Could you check a few things on this model? Use its own coordinates, in mm. Face numbers are marked on the shaded views. A direction names the side the tool comes from. Give positions to 0.01 mm unless a question says otherwise; leave off trailing zeros. Loops run counter-clockwise (first coordinate to the right, second up) from the corner with the lowest first, then second, coordinate; pieces in that order, holes last. Notation, with made-up numbers: (10, 19) - (29, 19) arc R17 cw to (29, 35) - close; hole circle Ø3 at (1.25, 63). An arc over 180 degrees is marked (long way). Write each question's results on one line, items separated by ' | '. Start each with the question number.
1) I want a section at B-B, the plane z = 0. Write out the boundary of the cut face in (x, y), and give its area (3 significant figures).
2) I want a section at D-D, the plane y = -378. Write out the boundary of the cut face in (x, z).
3) I want a section at A-A, the plane y = 0. Write out the boundary of the cut face in (x, z).
4) On a 3-axis mill with a long thin cutter (end or side, diameter ignored), from which of +Z, -Z, +X, -X, +Y, -Y can I reach the whole of each face in a straight line? I mean the marked faces 1, 2, 3 and 4. Say none if no direction works.
5) I want a section at C-C, the plane y = 365. Write out the boundary of the cut face in (x, z).
6) If I drill on probe 1 along Z at (x, y) = (199, 0); probe 2 along Y at (x, z) = (177, 71); probe 3 along Z at (x, y) = (140.5, -277.5), over which ranges is the centre line in solid material (lowest first)? Write a range as [from, to].
7) I'm going to push flat-ended pins straight in: pin 1 (3 mm diameter, centred on x = 171.5, z = -234, fed in from +Y); pin 2 (2 mm diameter, centred on x = 47, z = -451, fed in from -Y); pin 3 (1.5 mm diameter, centred on x = 141.5, z = 200, fed in from +Y); pin 4 (8 mm diameter, centred on y = 408, z = -248.5, fed in from -X). Where does each tip first touch, or does it pass through?
8) If we mould it in two halves opening along Y, with no side actions, what happens to the marked faces 5, 6, 7 and 8? For each: +Y half, -Y half, draft (parallel to the pull), parting line (faces both ways), or undercut.
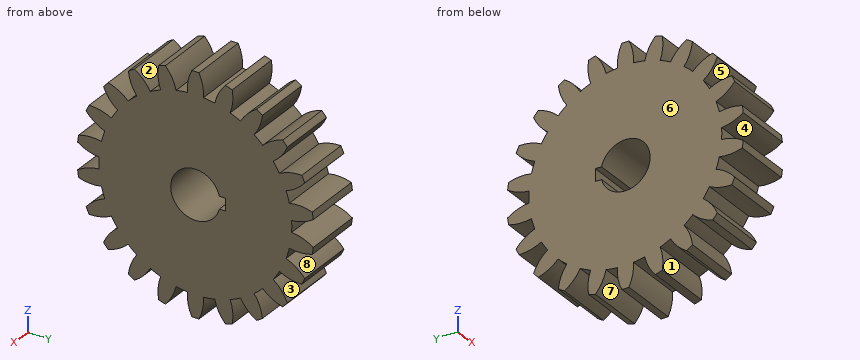
from build123d import *

# Parameters (mm, degrees)
BASPROSKE_W     = 304.8
BASPROSKE_H     = 609.6
TOOTHCUT_DEPTH  = 915.4
TEETHCUTS_COUNT = 22
TEETHCUTS_ANGLE = 343.636363636
BORSKE_R        = 127
BORE_DEPTH      = 304.8000508
KEYSKE_W        = 63.5
KEYSKE_H        = 154.8384
KEYWAY_DEPTH    = 304.8000508


with BuildPart() as part:
    # BasProSke → Base-Revolve (revolve)
    with BuildSketch(Plane(origin=(0, 0, 0), x_dir=(1, 0, 0), z_dir=(0, 1, 0)), mode=Mode.PRIVATE) as base_revolve_sk:
        with Locations((152.4, 304.8)):
            Rectangle(BASPROSKE_W, BASPROSKE_H)
    revolve(base_revolve_sk.sketch.rotate(Axis((-10, 0, 0), (1, 0, 0)), 180), axis=Axis((-10, 0, 0), (1, 0, 0)))

    # TooCutSke → ToothCut (cut, through all)
    with BuildSketch(Plane(origin=(0, 0, 0), x_dir=(0, 0, -1), z_dir=(1, 0, 0))):
        with BuildLine():
            ThreePointArc((29.477931626, 494.420755518), (0, 495.29873), (-29.477931626, 494.420755518))
            ThreePointArc((-29.477931626, 494.420755518), (-41.591539093, 552.716510617), (-68.665781689, 605.74593581))
            ThreePointArc((-68.665781689, 605.74593581), (0, 609.6254), (68.665781689, 605.74593581))
            ThreePointArc((68.665781689, 605.74593581), (41.591539093, 552.716510617), (29.477931626, 494.420755518))
        make_face()
    toothcut = extrude(amount=TOOTHCUT_DEPTH, mode=Mode.SUBTRACT)

    # TeethCuts: ToothCut ×22 about axis
    teethcuts_axis = Axis((-10, 0, 0), (1, 0, 0))
    for i in range(1, TEETHCUTS_COUNT):
        add(toothcut.rotate(teethcuts_axis, i * TEETHCUTS_ANGLE / (TEETHCUTS_COUNT - 1)), mode=Mode.SUBTRACT)

    # BorSke → Bore (cut, symmetric)
    with BuildSketch(Plane(origin=(0, 0, 0), x_dir=(0, 0, -1), z_dir=(1, 0, 0))):
        with Locations(Location((0, 0, 0), (0, 0, 180))):
            Circle(BORSKE_R)
    extrude(amount=BORE_DEPTH, both=True, mode=Mode.SUBTRACT)

    # KeySke → Keyway (cut, symmetric)
    with BuildSketch(Plane(origin=(0, 0, 0), x_dir=(0, 0, -1), z_dir=(1, 0, 0))):
        with Locations((0, 77.4192)):
            Rectangle(KEYSKE_W, KEYSKE_H)
    extrude(amount=KEYWAY_DEPTH, both=True, mode=Mode.SUBTRACT)


solid = part.part
Answers:
1) outline: (0, -495.3) - (304.8, -495.3) - (304.8, -127) - (0, -127) - close; (0, 154.84) - (304.8, 154.84) - (304.8, 495.3) - (0, 495.3) - close | area: 216,000 mm2
2) outline: (0, -380.86) - (304.8, -380.86) - (304.8, 380.86) - (0, 380.86) - close
3) outline: (0, -609.6) - (304.8, -609.6) - (304.8, -127) - (0, -127) - close; (0, 127) - (304.8, 127) - (304.8, 609.6) - (0, 609.6) - close
4) face 1: +X, -X | face 2: +Z, +X, -X | face 3: +X, -X, +Y | face 4: +X, -X, -Y
5) outline: (0, -371.26) - (304.8, -371.26) - (304.8, 371.26) - (0, 371.26) - close
6) probe 1: z = [-609.6, -127], [127, 609.6] | probe 2: y = [-605.45, -105.3], [105.3, 605.45] | probe 3: z = [-495.29, 495.29]
7) pin 1: stops at y = 561.02 | pin 2: stops at y = -333.16 | pin 3: stops at y = 525.45 | pin 4: stops at x = 0
8) face 5: -Y half | face 6: draft | face 7: undercut | face 8: +Y half
